from build123d import *

# Parameters (mm, degrees)
EXTRUDE_1_DEPTH     = 5
FILLET_1_R          = 2.5
FILLET_2_R          = 1
EXTRUDE_2_DEPTH     = 8
FILLET_3_R          = 2.5
SKETCH_5_W          = 1.467751534
SKETCH_5_H          = 4.178210798
SKETCH_5_W_2        = 1.389566385
CUT_EXTRUDE_1_DEPTH = 20
EXTRUDE_START       = 3
EXTRUDE_3_DEPTH     = 3
FILLET_4_R          = 2.5


with BuildPart() as part:
    # 草图1 → 凸台-拉伸1 (new body)
    with BuildSketch(Plane.XY):
        with BuildLine():
            Line((0, 0), (0, 28))
            Line((0, 28), (4, 28))
            Line((4, 28), (7.380946094, 20.749537704))
            Line((7.380946094, 20.749537704), (11.912485029, 22.862629012))
            Line((11.912485029, 22.862629012), (7.185351304, 33))
            Line((7.185351304, 33), (-5, 33))
            Line((-5, 33), (-5, -12))
            ThreePointArc((-5, -12), (-15, -22), (-25, -12))
            Line((-25, -12), (-25, -7))
            Line((-25, -7), (-30, -7))
            Line((-30, -7), (-30, -12))
            ThreePointArc((-30, -12), (-15, -27), (0, -12))
            Line((0, -12), (0, -5))
            Line((0, -5), (8, -5))
            Line((8, -5), (8, 0))
            Line((8, 0), (0, 0))
        make_face()
    extrude(amount=EXTRUDE_1_DEPTH)

    # 圆角1
    fillet_1_edges = [part.edges().sort_by_distance(p)[0] for p in [
        (9.646715562, 21.806083358, 0),
        (9.646715562, 21.806083358, 5),
        (7.185351304, 33, 2.5),
        (11.912485029, 22.862629012, 2.5),
        (7.380946094, 20.749537704, 2.5),
    ]]
    fillet(fillet_1_edges, radius=FILLET_1_R - 0.0001)  # a hair under: the kernel refuses the full size

    # 圆角2
    fillet_2_edges = [part.edges().sort_by_distance(p)[0] for p in [
        (-5, 33, 2.5),
    ]]
    fillet(fillet_2_edges, radius=FILLET_2_R)

    # 草图3 → 凸台-拉伸2 (add)
    with BuildSketch(Plane(origin=(0, 0, 0), x_dir=(0, 0, -1), z_dir=(1, 0, 0))):
        with BuildLine():
            Line((-5, 0), (0, 0))
            ThreePointArc((0, 0), (-2.5, 2.5), (-5, 0))
        make_face()
    extrude(amount=EXTRUDE_2_DEPTH)

    # 圆角3
    fillet_3_edges = [part.edges().sort_by_distance(p)[0] for p in [
        (8, -2.5, 0),
        (8, -5, 2.5),
        (8, -2.5, 5),
        (8, 2.5, 2.5),
    ]]
    fillet(fillet_3_edges, radius=FILLET_3_R - 0.0001)  # a hair under: the kernel refuses the full size

    # 草图4 → 旋转3 (revolve)
    with BuildSketch(Plane(origin=(4.4, 0, 0), x_dir=(0, 0, -1), z_dir=(1, 0, 0))):
        with BuildLine():
            Line((-5.5, 0), (0.5, 0))
            ThreePointArc((0.5, 0), (-2.5, 3), (-5.5, 0))
        make_face()
    revolve(axis=Axis((4.4, 0, 2.5), (0, 0, -1)))

    # 草图5 → 切除-拉伸1 (cut)
    with BuildSketch(Plane.ZY.offset(5)):
        with Locations((-0.733875767, -0.010051234)):
            Rectangle(SKETCH_5_W, SKETCH_5_H)
        with Locations((5.694783193, -0.010051234)):
            Rectangle(SKETCH_5_W_2, SKETCH_5_H)
    extrude(amount=-CUT_EXTRUDE_1_DEPTH, mode=Mode.SUBTRACT)

    # 草图6 → 凸台-拉伸3 (add)
    with BuildSketch(Plane(origin=(0, 0, 0), x_dir=(-1, 0, 0), z_dir=(0, 0, -1)).offset(EXTRUDE_START)):
        with BuildLine():
            Line((25, -7), (30, -7))
            Line((30, -7), (30, -12))
            ThreePointArc((30, -12), (15, -27), (0, -12))
            Line((0, -12), (5, -12))
            ThreePointArc((5, -12), (15, -22), (25, -12))
            Line((25, -12), (25, -7))
        make_face()
    extrude(amount=-EXTRUDE_3_DEPTH)

    # 圆角4
    fillet_4_edges = [part.edges().sort_by_distance(p)[0] for p in [
        (-2.5, -12, 0),
        (-27.5, -7, -3),
        (-30, -7, 1),
        (-25, -7, 1),
        (-27.5, -7, 5),
    ]]
    fillet(fillet_4_edges, radius=FILLET_4_R - 0.0001)  # a hair under: the kernel refuses the full size


solid = part.part
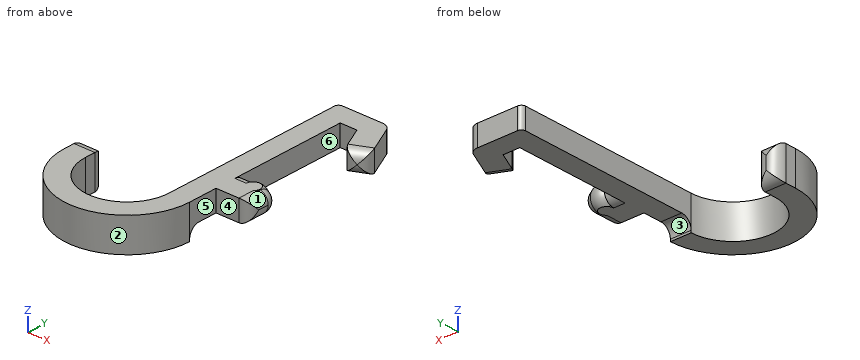
The listing builds one solid part. Answer for the finished solid, in the listing's coordinates (mm). Face numbers are marked on the shaded views. A direction names the side the tool comes from. Give positions to 0.01 mm unless a question says otherwise; leave off trailing zeros. Write each loop counter-clockwise with the first axis right and the second up, starting at its lowest first coordinate (ties: lowest second). Pieces come first, ordered by that corner, then holes.
Item 1: Find the intervals of material crossed by line 1 along X through (y, z) = (-10, 4.5); line 2 along Z through (x, y) = (-0.5, 11.5); line 3 along X through (y, z) = (-20.5, -1.25), in increasing order.
Item 2: Which of the six approach directions +Z, -Z, +X, -X, +Y, -Y give full straight-line access (tool end or side, diameter ignored) to the marked faces 1, 2 and 3?
Item 3: Flat-ended cylindrical pins translate along their axes: P1, Ø2, axis at x = -8.5, z = -1.5, coming from the -Y side; P2, Ø2, axis at y = -9, z = 0, coming from the +X side; P3, Ø2, axis at y = 19, z = 2.5, coming from the -X side. Find the tip coordinate at first contact, or state that the pin passes through.
Item 4: Section B-B, the plane z = -1.5 is taken. Write down the section's boundary in (x, y).
Item 5: Section D-D, the plane y = -6 is taken. Write down the section's boundary in (x, z), plus the area to 3 significant figures.
Item 6: Section C-C, the plane x = -15 is taken. Write down the section's boundary in (y, z).
Item 7: Determine the mould class of the marked faces 4, 5 and 6 for opening direction X: released by +X, released by -X, zero draft, split by the parting line, or undercut.
Item 8: Section A-A, the plane y = -15 is taken. Write down the section's boundary in (x, z), plus the area to 3 significant figures.
Completed:
1. line 1: x = -30 to -25, -5 to 0
1. line 2: z = 0 to 5
1. line 3: x = -27.36 to -20.27, -9.73 to -2.64
2. face 1: +Z, +X, -Y
2. face 2: +Z, -Z, -Y
2. face 3: -Z, +X, +Y
3. P1: stops at y = -25.96
3. P2: stops at x = 0
3. P3: stops at x = -5
4. outline: (-30, -12) arc R15 ccw to (0, -12) - (0, -11.79) - (-5, -11.79) - (-5, -12) arc R10 cw to (-25, -12) - (-25, -9.5) arc R2.5 ccw to (-26.5, -7.21) - (-28.5, -7.21) arc R2.5 ccw to (-30, -9.5) - close
5. outline: (-5, 0) - (0, 0) - (0, 5) - (-5, 5) - close
5. area: 25.0 mm2
6. outline: (-27, -3) - (-22, -3) - (-22, 5) - (-27, 5) - close
7. face 4: zero draft
7. face 5: released by +X
7. face 6: undercut
8. outline: (-29.7, -3) - (-24.54, -3) - (-24.54, 5) - (-29.7, 5) - close; (-5.46, -3) - (-0.3, -3) - (-0.3, 5) - (-5.46, 5) - close
8. area: 82.5 mm2
